from build123d import *

# Parameters (mm, degrees)
SKETCH1_W           = 251.46
SKETCH1_H           = 33.02
BOSS_EXTRUDE1_DEPTH = 3.175
CUT_EXTRUDE1_DEPTH  = 7.35
SKETCH3_W           = 190.412642411
SKETCH3_H           = 12.967021693
BOSS_EXTRUDE2_DEPTH = 6.35
SKETCH5_R           = 1.2573
CUT_EXTRUDE2_DEPTH  = 7.35
SKETCH6_W           = 4.445
SKETCH6_H           = 10.16
CUT_EXTRUDE4_DEPTH  = 7.35


with BuildPart() as part:
    # Sketch1 → Boss-Extrude1 (new body, symmetric)
    with BuildSketch(Plane(origin=(0, 0, 0), x_dir=(1, 0, 0), z_dir=(0, 1, 0))):
        Rectangle(SKETCH1_W, SKETCH1_H)
    extrude(amount=BOSS_EXTRUDE1_DEPTH, both=True)

    # Sketch2 → Cut-Extrude1 (cut, through all)
    with BuildSketch(Plane.XZ.offset(3.175)):
        Polygon((-96.266, -16.51), (-125.73, 12.954), (-125.73, -16.51), align=None)
    extrude(amount=-CUT_EXTRUDE1_DEPTH, mode=Mode.SUBTRACT)

    # Sketch3 → Boss-Extrude2 (add)
    with BuildSketch(Plane(origin=(0, 3.175, 0), x_dir=(1, 0, 0), z_dir=(0, 1, 0))):
        with Locations((1.633403272, -22.993510847)):
            Rectangle(SKETCH3_W, SKETCH3_H)
    extrude(amount=-BOSS_EXTRUDE2_DEPTH)

    # Sketch5 → Cut-Extrude2 (cut, through all)
    with BuildSketch(Plane(origin=(0, 3.175, 0), x_dir=(1, 0, 0), z_dir=(0, 1, 0))):
        with Locations((112.3696, 5.2324)):
            Circle(SKETCH5_R)
        with Locations((22.098, -16.51)):
            Circle(SKETCH5_R)
        with Locations((-51.2064, 1.524)):
            Circle(SKETCH5_R)
    extrude(amount=-CUT_EXTRUDE2_DEPTH, mode=Mode.SUBTRACT)

    # Sketch6 → Cut-Extrude4 (cut, through all)
    with BuildSketch(Plane.XZ.offset(3.175)):
        with Locations((86.8045, 7.721036343)):
            Rectangle(SKETCH6_W, SKETCH6_H)
        with Locations((118.4275, 7.721036343)):
            Rectangle(SKETCH6_W, SKETCH6_H)
        with Locations((102.616, -7.518963657)):
            Rectangle(SKETCH6_W, SKETCH6_H)
        with Locations((69.215, -7.518963657)):
            Rectangle(SKETCH6_W, SKETCH6_H)
        with Locations((-11.43, -7.518963657)):
            Rectangle(SKETCH6_W, SKETCH6_H)
        with Locations((-92.075, -7.518963657)):
            Rectangle(SKETCH6_W, SKETCH6_H)
    extrude(amount=-CUT_EXTRUDE4_DEPTH, mode=Mode.SUBTRACT)


solid = part.part
CAD build for the part. Positions are in the model's coordinates, mm. A direction names the side the tool comes from. Round coordinates to 2 decimals unless told otherwise and drop trailing zeros. Write each loop counter-clockwise with the first axis right and the second up, starting at its lowest first coordinate (ties: lowest second). Pieces come first, ordered by that corner, then holes. Notation, with made-up numbers: (26.5, -32) -> (42.5, -32) arc R26 cw to (42.5, -4) -> close; hole circle Ø2 at (-23, 54.5). An arc over 180 degrees is marked (long way). Answer as a JSON object with one key per item and string values.
(1) Which spindle directions (+Z, -Z, +X, -X, +Y, -Y) get a long thin tool onto all of the face, cutting with end or side? Do faces 1 (the face through (-92, 0, -12.599)), 2 (the face through (-110.792, -0.044, -1.984)), 3 (the face through (-93.573, 0, 23)), 4 (the face through (96.84, 0, 23)), 5 (the face through (13, 0, -16.51)). Say none if no direction does.
Reported:
{"face 1": "+Y, -Y", "face 2": "-Z, -X, +Y, -Y", "face 3": "+Z, -X, +Y, -Y", "face 4": "+Z, +X, +Y, -Y", "face 5": "-Z, +X, -X, +Y, -Y"}
(2) Band-saw the part on C-C, the plane y = 0.5. Count the separate pieces of the cut face and the enclosed holes in it, then the cut area to 3 significant figures.
Reported:
{"separate pieces": "1", "enclosed holes": "9", "area": "10,100 mm^2"}
(3) Two-plate mould, pull along X, no slides. Class faces 6 (the face through (0, 0, 29.477)), 7 (the face through (103, 0, -12.599)), 8 (the face through (125.73, 0, 0)): +X half, -X half, draft (parallel to the pull), parting line (faces both ways), or undercut.
Reported:
{"face 6": "draft", "face 7": "undercut", "face 8": "+X half"}
(4) Band-saw the part on B-B, the plane z = 26.5. List the corners of the cut face in (x, y) (3 decimals), then the cut area to 3 significant figures.
Reported:
{"outline": "(-93.573, -3.175) -> (96.84, -3.175) -> (96.84, 3.175) -> (-93.573, 3.175) -> close", "area": "1,210 mm^2"}
(5) Band-saw the part on A-A, the plane z = 5.5. List the corners of the cut face in (x, y) (3 decimals), then the cut area to 3 significant figures.
Reported:
{"outline": "(-118.276, -3.175) -> (84.582, -3.175) -> (84.582, 3.175) -> (-118.276, 3.175) -> close; (89.027, -3.175) -> (116.205, -3.175) -> (116.205, 3.175) -> (89.027, 3.175) -> close; (120.65, -3.175) -> (125.73, -3.175) -> (125.73, 3.175) -> (120.65, 3.175) -> close", "area": "1,490 mm^2"}
(6) Probe probe 1 along X at (y, z) = (-0.5, -4.5); probe 2 along X at (y, z) = (2.5, -7.5); probe 3 along Z at (x, y) = (67.5, -0.5). List the from-to ranges inside material, lowest first. Write a range as [from, to].
Reported:
{"probe 1": "x = [-108.28, -94.3], [-89.85, -13.65], [-9.21, 66.99], [71.44, 100.39], [104.84, 111.35], [113.39, 125.73]", "probe 2": "x = [-105.28, -94.3], [-89.85, -13.65], [-9.21, 66.99], [71.44, 100.39], [104.84, 125.73]", "probe 3": "z = [-16.51, -12.6], [-2.44, 29.48]"}
(7) Pin check, flat tips, straight feed: P1, Ø1.9, axis at y = 1, z = -6, coming from the -X side; P2, Ø1.9, axis at y = -1, z = 9.5, coming from the -X side; P3, Ø1.9, axis at y = 0.5, z = -5.5, coming from the -X side. Stop position of each tip, or through.
Reported:
{"P1": "stops at x = -107.73", "P2": "stops at x = -123.23", "P3": "stops at x = -108.23"}
